```python
from build123d import *

# Parameters (mm, degrees)
SKETCH1_R                 = 18
BOSS_EXTRUDE1_DEPTH       = 38
BOSS_EXTRUDE2_DEPTH       = 16
BOSS_EXTRUDE2_DEPTH_BACK  = 45
SKETCH2_R                 = 2.5
SKETCH3_R                 = 7
BOSS_EXTRUDE3_DEPTH       = 4
M3X0_5_TAPPED_HOLE1_D     = 2.5
M3X0_5_TAPPED_HOLE1_DEPTH = 3
M3X0_5_TAPPED_HOLE1_TIP   = 0.751075774
SKETCH6_R                 = 2.5
CUT_EXTRUDE1_DEPTH        = 1.25
CUT_EXTRUDE2_START        = -1.6
SKETCH7_R                 = 18
SKETCH7_R_2               = 16.635
CUT_EXTRUDE2_DEPTH        = 1.6
FILLET1_R                 = 0.75


with BuildPart() as part:
    # Sketch1 → Boss-Extrude1 (new body)
    with BuildSketch(Plane.XY):
        Circle(SKETCH1_R)
    extrude(amount=BOSS_EXTRUDE1_DEPTH)

    # Sketch2 → Boss-Extrude2 (add, two sides: drawn at the far end of the back side and taken through both)
    with BuildSketch(Plane(origin=(0, 0, 0), x_dir=(-1, 0, 0), z_dir=(0, 0, -1)).offset(-BOSS_EXTRUDE2_DEPTH_BACK)):
        Circle(SKETCH2_R)
    extrude(amount=BOSS_EXTRUDE2_DEPTH + BOSS_EXTRUDE2_DEPTH_BACK)

    # Sketch3 → Boss-Extrude3 (add)
    with BuildSketch(Plane(origin=(0, 0, 0), x_dir=(-1, 0, 0), z_dir=(0, 0, -1))):
        with Locations(Location((0, 0, 0), (0, 0, 180))):
            Circle(SKETCH3_R)
    boss_extrude3 = extrude(amount=BOSS_EXTRUDE3_DEPTH)

    # M3x0.5 Tapped Hole1
    with Locations(Plane(origin=(0, 0, 0), x_dir=(-1, 0, 0), z_dir=(0, 0, -1))):
        with Locations((0, 12.5), (-10.825317547, 6.25), (0, -12.5), (10.825317547, 6.25)):
            Hole(M3X0_5_TAPPED_HOLE1_D / 2, depth=M3X0_5_TAPPED_HOLE1_DEPTH)
            with Locations((0, 0, -(M3X0_5_TAPPED_HOLE1_DEPTH + M3X0_5_TAPPED_HOLE1_TIP / 2))):  # 118° drill point
                Cone(0, M3X0_5_TAPPED_HOLE1_D / 2, M3X0_5_TAPPED_HOLE1_TIP, mode=Mode.SUBTRACT)

    # Sketch6 → Cut-Extrude1 (cut)
    with BuildSketch(Plane.XY.offset(45)):
        with Locations(Location((0, 0, 0), (0, 0, 180))):
            Circle(SKETCH6_R)
    extrude(amount=-CUT_EXTRUDE1_DEPTH, mode=Mode.SUBTRACT)

    # Mirror1: Boss-Extrude3 across plane
    add(boss_extrude3.mirror(Plane(origin=(0, 0, 19), x_dir=(1, 0, 0), z_dir=(0, 0, -1))))

    # Sketch7 → Cut-Extrude2 (cut)
    with BuildSketch(Plane.XY.offset(38).offset(CUT_EXTRUDE2_START)):
        Circle(SKETCH7_R)
        Circle(SKETCH7_R_2, mode=Mode.SUBTRACT)
    extrude(amount=CUT_EXTRUDE2_DEPTH, mode=Mode.SUBTRACT)

    # Fillet1
    fillet1_edges = [part.edges().sort_by_distance(p)[0] for p in [
        (-16.635, 0, 38),
    ]]
    fillet(fillet1_edges, radius=FILLET1_R)

    # Sketch8 → Cut-Revolve1 (revolve, cut)
    with BuildSketch(Plane(origin=(0, 0, 0), x_dir=(1, 0, 0), z_dir=(0, 1, 0)), mode=Mode.PRIVATE) as cut_revolve1_sk:
        Polygon((2.5, 16), (2.5, 14.4125), (2.4238, 16), align=None)
    revolve(cut_revolve1_sk.sketch.rotate(Axis((0, 0, -16), (0, 0, -1)), 180), axis=Axis((0, 0, -16), (0, 0, -1)), mode=Mode.SUBTRACT)


solid = part.part
```
Can you work these out from the model? Positions are in its coordinate system, mm. A direction names the side the tool comes from. Round coordinates to 2 decimals unless told otherwise and drop trailing zeros. Order: outer loops, then holes, each group sorted by start corner. A loop starts at its lowest first (then second) coordinate and runs counter-clockwise, first axis right, second up. Notation, with made-up numbers: (-25, 58) -> (5, 58) arc R34 cw to (5, 88) -> close; hole circle Ø4 at (-35.5, -20). An arc over 180 degrees is marked (long way). Return JSON: item names as keys, results as strings. Group by question number.
1. If we section it at B-B, the plane z = 39: Write out the boundary of the cut face in (x, y), then the cut area to 3 significant figures.
2. I need wall thicknesses on line 1 (Y direction, x = 0, z = 2.2); line 2 (X direction, y = 6.25, z = 1.75); line 3 (Z direction, x = -7, y = -15.5). Which ranges of each line are inside material? Lowest first, please. Write a range as [from, to].
3. We'd pull the mould along Y, two halves only. Please class faces 4 (the face through (15.367, -6.371, 36.819)), 5 (the face through (-0.2, 12.42, 3.62)), 6 (the face through (3, 0, 42)): released by +Y, released by -Y, zero draft, split by the parting line, or undercut.
4. Will these pins go through, and if not, where does the flat tip stop? pin 1 (8 mm diameter, centred on x = -3, z = 27.5, fed in from -Y); pin 2 (12 mm diameter, centred on x = -4, z = 0, fed in from +Y); pin 3 (8 mm diameter, centred on y = 9, z = 27, fed in from +X).
5. Which directions (+Z, -Z, +X, -X, +Y, -Y) give clear straight access to the entire face, cutting with the end or side of a thin tool? Please do faces 1 (the face through (0, 0, -16)), 2 (the face through (12, -12, 36.4)), 3 (the face through (3, 0, -4)).
Output values:
{
 "1": {"outline": "circle Ø14 at (0, 0)", "area": "154 mm²"},
 "2": {"line 1": "[-18, -13.75], [-11.25, 11.25], [13.75, 18]", "line 2": "[-16.88, -12.08], [-9.58, 9.58], [12.08, 16.88]", "line 3": "[0, 36.4]"},
 "3": {"face 4": "split by the parting line", "face 5": "undercut", "face 6": "zero draft"},
 "4": {"pin 1": "y = -18", "pin 2": "y = 18", "pin 3": "x = 17.29"},
 "5": {"face 1": "-Z, +X, -X, +Y, -Y", "face 2": "+Z", "face 3": "-Z"}
}
